Drawing for the job (mm, zero at the part's lowest x, y, z). A direction names the side the tool comes from. Round coordinates to 2 decimals unless told otherwise and drop trailing zeros. Write each loop counter-clockwise with the first axis right and the second up, starting at its lowest first coordinate (ties: lowest second). Pieces come first, ordered by that corner, then holes. Notation, with made-up numbers: (30.5, 88.5) - (83.5, 88.5) arc R20 cw to (83.5, 116.5) - close; hole circle Ø4 at (-28.75, 60). An arc over 180 degrees is marked (long way). One line per question, with ' | ' between items.
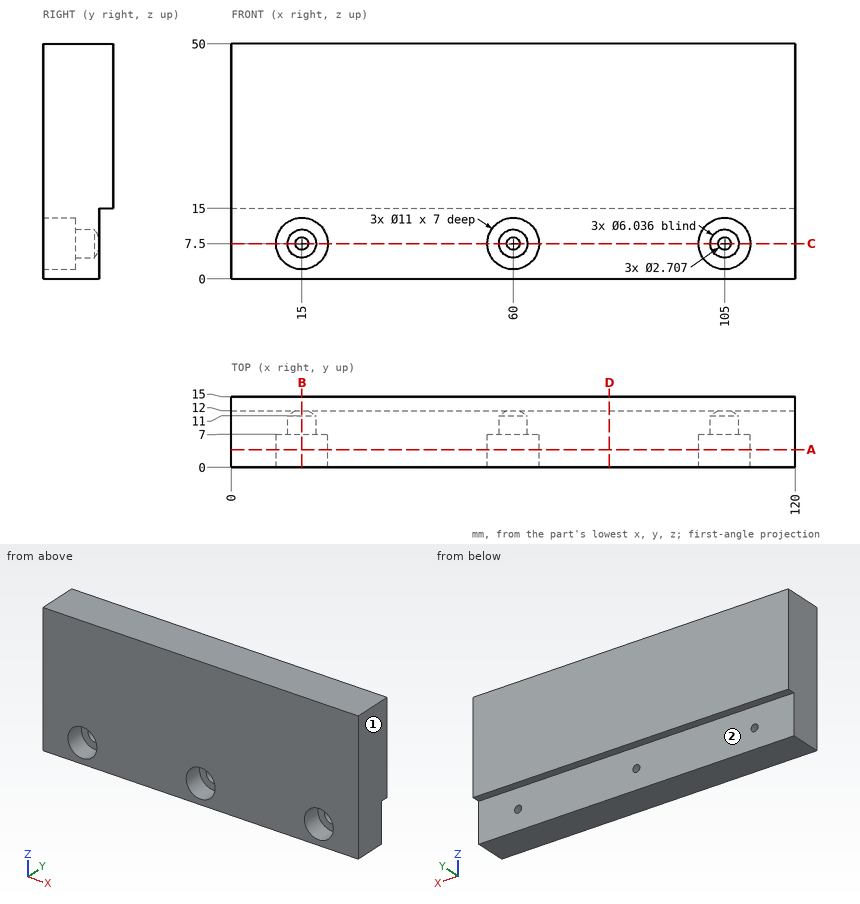
Q1. Which spindle directions (+Z, -Z, +X, -X, +Y, -Y) get a long thin tool onto all of the face, cutting with end or side? Do the marked faces 1 and 2. Say none if no direction does.
Found:
face 1: +Z, -Z, +X, +Y, -Y | face 2: -Z, +X, -X, +Y
Q2. Saw through at C-C, the plane z = 7.5. State how many separate pieces and enclosed holes the cut face has, then the cut area to 3 significant figures.
Found:
separate pieces: 4 | enclosed holes: 0 | area: 1,120 mm^2
Q3. Saw through at A-A, the plane y = 3.75. List the corners of the cut face in (x, z).
Found:
outline: (0, 0) - (120, 0) - (120, 50) - (0, 50) - close; hole circle Ø11 at (15, 7.5); hole circle Ø11 at (60, 7.5); hole circle Ø11 at (105, 7.5)
Q4. Drill centre lines: L1, parallel to X at y = 2, z = 7.5; L2, parallel to Z at x = 105, y = 9.05; L3, parallel to Z at x = 105, y = 4.5. Where is each one in solid material? Low to high. Write a range as from..to.
Found:
L1: 0..9.5, 20.5..54.5, 65.5..99.5, 110.5..120 | L2: 0..4.48, 10.52..50 | L3: 0..2, 13..50
Q5. Saw through at B-B, the plane x = 15. List the corners of the cut face in (y, z).
Found:
outline: (0, 0) - (12, 0) - (12, 6.15) - (11, 4.48) - (7, 4.48) - (7, 2) - (0, 2) - close; (0, 13) - (7, 13) - (7, 10.52) - (11, 10.52) - (12, 8.85) - (12, 15) - (15, 15) - (15, 50) - (0, 50) - close
Q6. Saw through at D-D, the plane x = 80.5. List the corners of the cut face in (y, z).
Found:
outline: (0, 0) - (12, 0) - (12, 15) - (15, 15) - (15, 50) - (0, 50) - close
Q7. Drop flat-ended pins along their axis: pin 1 (9 mm diameter, centred on x = 105, z = 7.5, fed in from +Y); pin 2 (5.5 mm diameter, centred on x = 58, z = 9, fed in from -Y); pin 3 (5 mm diameter, centred on x = 105, z = 7.5, fed in from -Y). Give the stop position or say it passes through.
Found:
pin 1: y = 12 | pin 2: y = 7 | pin 3: y = 11.31
